Source: CAD feature listing. Evaluate the final solid. Frame: model axes, mm. A direction names the side the tool comes from. Round coordinates to 2 decimals unless told otherwise and drop trailing zeros. Order: outer loops, then holes, each group sorted by start corner. A loop starts at its lowest first (then second) coordinate and runs counter-clockwise, first axis right, second up. Notation, with made-up numbers: M 10.5,65 L 39.5,65 A7 cw 39.5,77 Z; hole C -39.5,41.5 d11. An arc over 180 degrees is marked long. Answer as CSV lines item,"result". Start each with the question number.
Item 1: Section query A-A on z = -2.5. Return the cut outline in (x, y), plus the area to 3 significant figures.
Item 2: Section query B-B on z = 7. Return the cut outline in (x, y), plus the area to 3 significant figures.
Item 3: Section query D-D on y = -1.75. Return the cut outline in (x, z), plus the area to 3 significant figures.
Item 4: Set-up query: faces 1 (the face through (4.453, 0, -1)), 2 (the face through (-1.081, 2.112, -6.437)), 3 (the face through (-0.503, -2.723, 4.437)). Return all of +Z, -Z, +X, -X, +Y, -Y with unobstructed straight access to the full face (end or side cutting, diameter ignored); none if empty.
Item 5: Pull-direction query (X, two-part tool) for faces 4 (the face through (-0.591, 2.576, 4.437)), 5 (the face through (-1, -1, -11)), 6 (the face through (-5.26, 4.63, -1.14)), 7 (the face through (-0.577, -0.082, -6.437)); classes: +X half, -X half, draft (parallel to the pull), parting line (faces both ways), or undercut.
Item 6: Line query: line 1 (Y direction, x = -0.5, z = 0.25); line 2 (Y direction, x = -1, z = 8); line 3 (X direction, y = -0.5, z = 6.5). Output: solid intervals per line, ascending. Write a range as [from, to].
Item 7: Section query C-C on x = 0.5. Return the cut outline in (y, z).
from build123d import *

# Parameters (mm, degrees)
F0_W     = 10
F0_H     = 10
F0_W_2   = 4
F0_H_2   = 0.3
F1_DEPTH = 9
F2_DEPTH = 2
F3_W     = 10
F3_H     = 10
F4_DEPTH = 9
F6_R     = 1


with BuildPart() as f1:
    # F0 (on Top) → F1 (new body)
    with BuildSketch(Plane.XY):
        with Locations((-0.546654, -0.073579)):
            Rectangle(F0_W, F0_H)
        with BuildLine():
            Line((1.453346, 0.076421), (1.453346, -0.223579))
            Line((1.453346, -0.223579), (1.453346, -0.723579))
            ThreePointArc((1.453346, -0.723579), (-0.546654, -2.723579), (-2.546654, -0.723579))
            Line((-2.546654, -0.723579), (-2.546654, -0.223579))
            Line((-2.546654, -0.223579), (-2.546654, 0.076421))
            Line((-2.546654, 0.076421), (-2.546654, 0.576421))
            ThreePointArc((-2.546654, 0.576421), (-0.546654, 2.576421), (1.453346, 0.576421))
            Line((1.453346, 0.576421), (1.453346, 0.076421))
        make_face(mode=Mode.SUBTRACT)
        with Locations((-0.546654, -0.073579)):
            Rectangle(F0_W_2, F0_H_2)
    extrude(amount=F1_DEPTH)

    # F0 (on Top) → F2 (join)
    with BuildSketch(Plane.XY):
        with Locations((-0.546654, -0.073579)):
            Rectangle(F0_W, F0_H)
        with BuildLine():
            Line((1.453346, 0.076421), (1.453346, -0.223579))
            Line((1.453346, -0.223579), (1.453346, -0.723579))
            ThreePointArc((1.453346, -0.723579), (-0.546654, -2.723579), (-2.546654, -0.723579))
            Line((-2.546654, -0.723579), (-2.546654, -0.223579))
            Line((-2.546654, -0.223579), (-2.546654, 0.076421))
            Line((-2.546654, 0.076421), (-2.546654, 0.576421))
            ThreePointArc((-2.546654, 0.576421), (-0.546654, 2.576421), (1.453346, 0.576421))
            Line((1.453346, 0.576421), (1.453346, 0.076421))
        make_face(mode=Mode.SUBTRACT)
        with BuildLine():
            Line((1.453346, -0.723579), (1.453346, -0.223579))
            Line((1.453346, -0.223579), (-2.546654, -0.223579))
            Line((-2.546654, -0.223579), (-2.546654, -0.723579))
            ThreePointArc((-2.546654, -0.723579), (-0.546654, -2.723579), (1.453346, -0.723579))
        make_face()
        with Locations((-0.546654, -0.073579)):
            Rectangle(F0_W_2, F0_H_2)
        with BuildLine():
            Line((-2.546654, 0.076421), (1.453346, 0.076421))
            Line((1.453346, 0.076421), (1.453346, 0.576421))
            ThreePointArc((1.453346, 0.576421), (-0.546654, 2.576421), (-2.546654, 0.576421))
            Line((-2.546654, 0.576421), (-2.546654, 0.076421))
        make_face()
    extrude(amount=-F2_DEPTH)


with BuildPart() as f4:
    # F3 (on face) → F4 (new body)
    with BuildSketch(Plane(origin=(0, 0, -2), x_dir=(1, 0, 0), z_dir=(0, 0, -1))):
        with Locations((-0.546654, 0.073579)):
            Rectangle(F3_W, F3_H)
        with BuildLine():
            ThreePointArc((-2.719987, 0.655922), (-0.25297, 2.30433), (1.703346, 0.073579))
            ThreePointArc((1.703346, 0.073579), (1.684097, -0.220104), (1.626679, -0.508763))
            ThreePointArc((1.626679, -0.508763), (-1.128997, -2.099754), (-2.719987, 0.655922))
        make_face(mode=Mode.SUBTRACT)
        with BuildLine():
            ThreePointArc((1.626679, -0.508763), (1.684097, -0.220104), (1.703346, 0.073579))
            ThreePointArc((1.703346, 0.073579), (-0.25297, 2.30433), (-2.719987, 0.655922))
            Line((-2.719987, 0.655922), (1.626679, -0.508763))
        make_face()
    extrude(amount=F4_DEPTH)


with BuildPart() as f1_1:
    add(f1.part)

    # F5: union F4
    add(f4.part)

    # F6
    f6_edges = [f1_1.edges().sort_by_distance(p)[0] for p in [
        (-5.546654, 4.926421, -1),
        (4.453346, 4.926421, -1),
        (4.453346, -5.073579, -1),
        (-5.546654, -5.073579, -1),
    ]]
    fillet(f6_edges, radius=F6_R)


solid = f1_1.part
Results:
1,outline,"M -5.55,-4.07 A1 ccw -4.55,-5.07 L 3.45,-5.07 A1 ccw 4.45,-4.07 L 4.45,3.93 A1 ccw 3.45,4.93 L -4.55,4.93 A1 ccw -5.55,3.93 Z; hole M -2.72,-0.66 L 1.63,0.51 A2.25 ccw Z"
1,area,"91.2 mm^2"
2,outline,"M -5.55,-4.07 A1 ccw -4.55,-5.07 L 3.45,-5.07 A1 ccw 4.45,-4.07 L 4.45,3.93 A1 ccw 3.45,4.93 L -4.55,4.93 A1 ccw -5.55,3.93 Z; hole M -2.55,-0.72 A2 ccw 1.45,-0.72 L 1.45,-0.22 L -2.55,-0.22 Z; hole M -2.55,0.08 L 1.45,0.08 L 1.45,0.58 A2 ccw -2.55,0.58 Z"
2,area,"82.6 mm^2"
3,outline,"M -5.55,-11 L 4.45,-11 L 4.45,9 L 1.17,9 L 1.17,0 L -2.26,0 L -2.26,9 L -5.55,9 Z"
3,area,"169 mm^2"
4,face 1,"+Z, -Z, +X, +Y, -Y"
4,face 2,"-Z"
4,face 3,"+Z"
5,face 4,"undercut"
5,face 5,"draft"
5,face 6,"-X half"
5,face 7,"undercut"
6,line 1,"[-5.07, -2.72], [-0.22, 0.08], [2.58, 4.93]"
6,line 2,"[-5.07, -2.67], [-0.22, 0.08], [2.52, 4.93]"
6,line 3,"[-5.55, -2.55], [1.45, 4.45]"
7,outline,"M -5.07,-11 L 0.21,-11 L 0.21,-2 L 1.92,-2 L 1.92,-11 L 4.93,-11 L 4.93,9 L 2.28,9 L 2.28,0 L 0.08,0 L 0.08,9 L -0.22,9 L -0.22,0 L -2.43,0 L -2.43,9 L -5.07,9 Z"
